The model under review builds one solid part; all positions refer to its coordinate system, in mm. Face numbers are marked on the shaded views. A direction names the side the tool comes from. Coordinates: 2 decimals unless noted, no trailing zeros. Write each loop counter-clockwise with the first axis right and the second up, starting at its lowest first coordinate (ties: lowest second). Pieces come first, ordered by that corner, then holes. Notation, with made-up numbers: M -21.5,-17 L -7.5,-17 A17 cw -7.5,-6 Z; hole C 64.25,5 d2. An arc over 180 degrees is marked long. Answer as a JSON object with one key per item and string values.
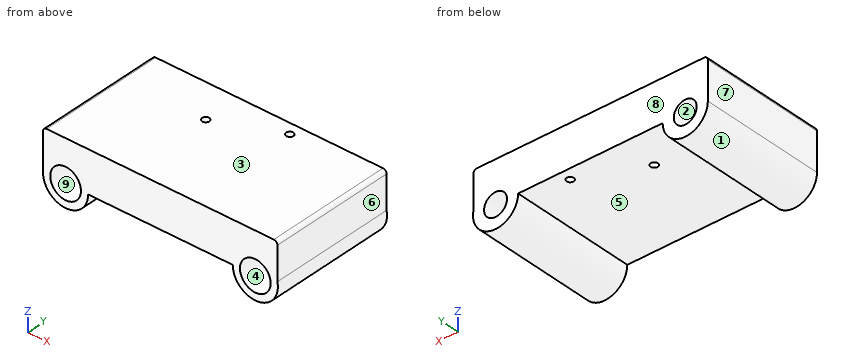
```python
from build123d import *

# Parameters (mm, degrees)
BOSS_EXTRUDE1_DEPTH = 35
SKETCH2_R           = 3.175
CUT_EXTRUDE1_DEPTH  = 36
SKETCH3_R           = 4.25
CUT_EXTRUDE2_DEPTH  = 9
SKETCH4_R           = 1
CUT_EXTRUDE4_DEPTH  = 18.75
FILLET1_R           = 1


with BuildPart() as part:
    # Sketch1 → Boss-Extrude1 (new body)
    with BuildSketch(Plane(origin=(0, 0, 0), x_dir=(1, 0, 0), z_dir=(0, 1, 0))):
        with BuildLine():
            Line((-24.985807588, 0), (15.020468055, 0))
            ThreePointArc((15.020468055, 0), (21.898649068, 6.218350956), (27.394192412, -1.25))
            Line((27.394192412, -1.25), (27.394192412, -11.5))
            Line((27.394192412, -11.5), (-37.485807588, -11.5))
            Line((-37.485807588, -11.5), (-37.485807588, 0))
            ThreePointArc((-37.485807588, 0), (-31.235807588, 6.25), (-24.985807588, 0))
        make_face()
    extrude(amount=BOSS_EXTRUDE1_DEPTH)

    # Sketch2 → Cut-Extrude1 (cut, through all)
    with BuildSketch(Plane(origin=(0, 35, 0), x_dir=(1, 0, 0), z_dir=(0, 1, 0))):
        with Locations((-31.235807588, 0)):
            Circle(SKETCH2_R)
        with Locations((21.270468055, 0)):
            Circle(SKETCH2_R)
    extrude(amount=-CUT_EXTRUDE1_DEPTH, mode=Mode.SUBTRACT)

    # Sketch3 → Cut-Extrude2 (cut)
    with BuildSketch(Plane.XZ):
        with Locations((21.270468055, 0)):
            Circle(SKETCH3_R)
        with Locations((-31.235807588, 0)):
            Circle(SKETCH3_R)
    extrude(amount=-CUT_EXTRUDE2_DEPTH, mode=Mode.SUBTRACT)

    # Sketch4 → Cut-Extrude4 (cut, through all)
    with BuildSketch(Plane.XY.offset(11.5)):
        with Locations((-13.485807588, 24.385)):
            Circle(SKETCH4_R)
        with Locations((3.394192412, 31.785)):
            Circle(SKETCH4_R)
    extrude(amount=-CUT_EXTRUDE4_DEPTH, mode=Mode.SUBTRACT)

    # Fillet1
    fillet1_edges = [part.edges().sort_by_distance(p)[0] for p in [
        (27.394192412, 17.5, 11.5),
        (-37.485807588, 17.5, 11.5),
    ]]
    fillet(fillet1_edges, radius=FILLET1_R)


solid = part.part
```
(1) Add section B-B on y = 22. Give the boundary of the cut face in (x, z) (3 decimals).
Results list:
{"outline": "M -37.486,0 A6.25 ccw -24.986,0 L 15.02,0 A6.25 ccw long 27.394,1.25 L 27.394,10.5 A1 ccw 26.394,11.5 L -36.486,11.5 A1 ccw -37.486,10.5 Z; hole C -31.236,0 d6.35; hole C 21.27,0 d6.35"}
(2) Add section A-A on y = 8. Give the boundary of the cut face in (x, z).
Results list:
{"outline": "M -37.49,0 A6.25 ccw -24.99,0 L 15.02,0 A6.25 ccw long 27.39,1.25 L 27.39,10.5 A1 ccw 26.39,11.5 L -36.49,11.5 A1 ccw -37.49,10.5 Z; hole C -31.24,0 d8.5; hole C 21.27,0 d8.5"}
(3) For the marked faces 5, 6, 7, 8 and 9, list the 3-axis set-ups (+Z, -Z, +X, -X, +Y, -Y) from which the entire face can be reached by the end or side of a thin tool; tool diameter is ignored.
Results list:
{"face 5": "-Z, +Y, -Y", "face 6": "+Z, +X, +Y, -Y", "face 7": "+Z, -Z, -X, +Y, -Y", "face 8": "+Z, -Z, +X, -X, +Y", "face 9": "-Y"}
(4) Draft analysis for pull direction Z (two halves, no side actions). For the marked faces 1, 2, 3 and 4, state which applies: released by +Z, released by -Z, zero draft, split by the parting line, or undercut.
Results list:
{"face 1": "released by -Z", "face 2": "undercut", "face 3": "released by +Z", "face 4": "undercut"}
(5) Add section C-C on x = -3. Give the boundary of the cut face in (y, z).
Results list:
{"outline": "M 0,0 L 35,0 L 35,11.5 L 0,11.5 Z"}
(6) For pin 1 Ø1.2 at (x, y) = (-13.49, 24.38) entering from +Z; pin 2 Ø7 at (x, z) = (21.27, 0) entering from -Y; pin 3 Ø3 at (x, y) = (6.5, 21.5) entering from -Z; pin 4 Ø1 at (y, z) = (19, -4.5) entering from -X, all flat-tipped, find the tip position at first contact; note any pin that passes through.
Results list:
{"pin 1": "through", "pin 2": "y = 9", "pin 3": "z = 0", "pin 4": "x = -36.04"}
(7) Wall thickness on line 1 along X through (y, z) = (33, 2.25); line 2 along X through (y, z) = (24.5, -1.5); line 3 along X through (y, z) = (19.5, -2.25): over which ranges is each line inside the solid? List them lowest first. Write a range as from..to.
Results list:
{"line 1": "-37.49..-33.48, -29..19.03, 23.51..27.39", "line 2": "-37.3..-34.03, -28.44..-25.17, 15.2..18.47, 24.07..27.34", "line 3": "-37.07..-33.48, -29..-25.4, 15.44..19.03, 23.51..27.1"}
